For this review, take the finished solid that the model builds, in its own axes (mm). Coordinates: 2 decimals unless noted, no trailing zeros. Loops run counter-clockwise (first coordinate to the right, second up) from the corner with the lowest first, then second, coordinate; pieces in that order, holes last. Notation, with made-up numbers: (66.5, -29.75) - (86.5, -29.75) arc R25 ccw to (86.5, -15.75) - close; hole circle Ø3 at (-4, 20.5). An arc over 180 degrees is marked (long way). Use one line per item in the form item = value. Start each with the question number.
1. Add section D-D on x = -187. Give the boundary of the cut face in (y, z).
2. Add section C-C on y = 0. Give the boundary of the cut face in (x, z), and give its area (3 significant figures).
3. To check wall thickness, follow probe 1 along Y at (x, z) = (240, 558); probe 2 along Z at (x, y) = (-128.5, 56). State the ranges of each line that lie inside material, in increasing order.
4. For pin 1 Ø15 at (x, z) = (244, 327.5) entering from +Y; pin 2 Ø25 at (y, z) = (307, -35.5) entering from +X; pin 3 Ø22.5 at (x, z) = (-18, -30) entering from -Y, all flat-tipped, find the tip position at first contact; note any pin that passes through.
5. Add section A-A on z = 254.5. Give the boundary of the cut face in (x, y).
6. Add section B-B on x = 0. Give the boundary of the cut face in (y, z), and give its area (4 significant figures).
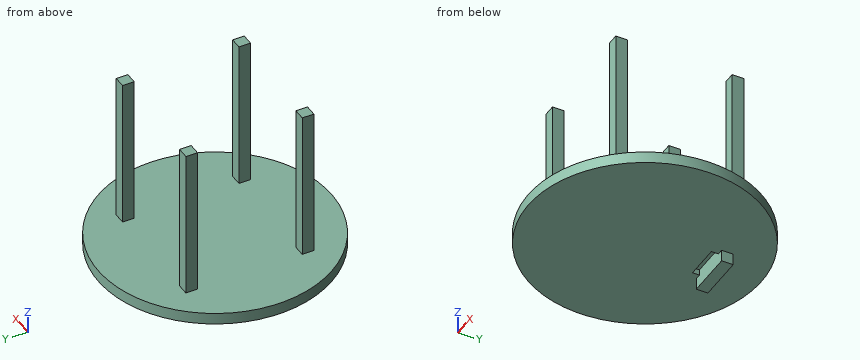
```python
from build123d import *

# Parameters (mm, degrees)
SKETCH_1_R          = 500
EXTRUDE_1_DEPTH     = 50
SKETCH_2_W          = 50
SKETCH_2_H          = 50
EXTRUDE_2_DEPTH     = 700
SKETCH_3_W          = 50
SKETCH_3_H          = 50
EXTRUDE_3_DEPTH     = 700
SKETCH_4_W          = 50
SKETCH_4_H          = 50
EXTRUDE_4_DEPTH     = 700
SKETCH_5_W          = 50
SKETCH_5_H          = 50
EXTRUDE_5_DEPTH     = 700
SKETCH_6_W          = 200
SKETCH_6_H          = 100
EXTRUDE_6_DEPTH     = 50
SKETCH_7_W          = 150
SKETCH_7_H          = 50
CUT_EXTRUDE_1_DEPTH = 30


with BuildPart() as part:
    # 草图1 → 凸台-拉伸1 (new body)
    with BuildSketch(Plane.XY):
        Circle(SKETCH_1_R)
    extrude(amount=EXTRUDE_1_DEPTH)

    # 草图2 → 凸台-拉伸2 (add)
    with BuildSketch(Plane.XY):
        with Locations((250, 250)):
            Rectangle(SKETCH_2_W, SKETCH_2_H)
    extrude(amount=EXTRUDE_2_DEPTH)

    # 草图3 → 凸台-拉伸3 (add)
    with BuildSketch(Plane.XY):
        with Locations((-250, 250)):
            Rectangle(SKETCH_3_W, SKETCH_3_H)
    extrude(amount=EXTRUDE_3_DEPTH)

    # 草图4 → 凸台-拉伸4 (add)
    with BuildSketch(Plane.XY):
        with Locations((250, -250)):
            Rectangle(SKETCH_4_W, SKETCH_4_H)
    extrude(amount=EXTRUDE_4_DEPTH)

    # 草图5 → 凸台-拉伸5 (add)
    with BuildSketch(Plane.XY):
        with Locations((-250, -250)):
            Rectangle(SKETCH_5_W, SKETCH_5_H)
    extrude(amount=EXTRUDE_5_DEPTH)

    # 草图6 → 凸台-拉伸6 (add)
    with BuildSketch(Plane(origin=(0, 275, 0), x_dir=(1, 0, 0), z_dir=(0, 1, 0))):
        Rectangle(SKETCH_6_W, SKETCH_6_H)
    extrude(amount=EXTRUDE_6_DEPTH)

    # 草图7 → 切除-拉伸1 (cut)
    with BuildSketch(Plane(origin=(0, 275, 0), x_dir=(1, 0, 0), z_dir=(0, 1, 0))):
        Rectangle(SKETCH_7_W, SKETCH_7_H)
    extrude(amount=-CUT_EXTRUDE_1_DEPTH, mode=Mode.SUBTRACT)


solid = part.part
```
Conclusion:
q1.outline = (-463.71, 0) - (463.71, 0) - (463.71, 50) - (-463.71, 50) - close
q2.outline = (-500, 0) - (500, 0) - (500, 50) - (-500, 50) - close
q2.area = 50,000 mm^2
q3.probe_1 = -275 to -225, 225 to 275
q3.probe_2 = 0 to 50
q4.pin_1 = 275
q4.pin_2 = 100
q4.pin_3 = 275
q5.outline = (-275, -275) - (-225, -275) - (-225, -225) - (-275, -225) - close; (-275, 225) - (-225, 225) - (-225, 275) - (-275, 275) - close; (225, -275) - (275, -275) - (275, -225) - (225, -225) - close; (225, 225) - (275, 225) - (275, 275) - (225, 275) - close
q6.outline = (-500, 0) - (245, 0) - (245, 25) - (275, 25) - (275, -50) - (325, -50) - (325, 0) - (500, 0) - (500, 50) - (-500, 50) - close
q6.area = 51,750 mm^2
